Check sheet for the drawn part. Datum: minimum x, y, z corner. Units: mm. Round coordinates to 2 decimals unless told otherwise and drop trailing zeros. Write each loop counter-clockwise with the first axis right and the second up, starting at its lowest first coordinate (ties: lowest second). Pieces come first, ordered by that corner, then holes. Notation, with made-up numbers: M -7.75,-14.5 L 30.25,-14.5 A23 cw 30.25,7.5 Z; hole C 6.5,-30 d11. An arc over 180 degrees is marked long. One line per item, written item: value.
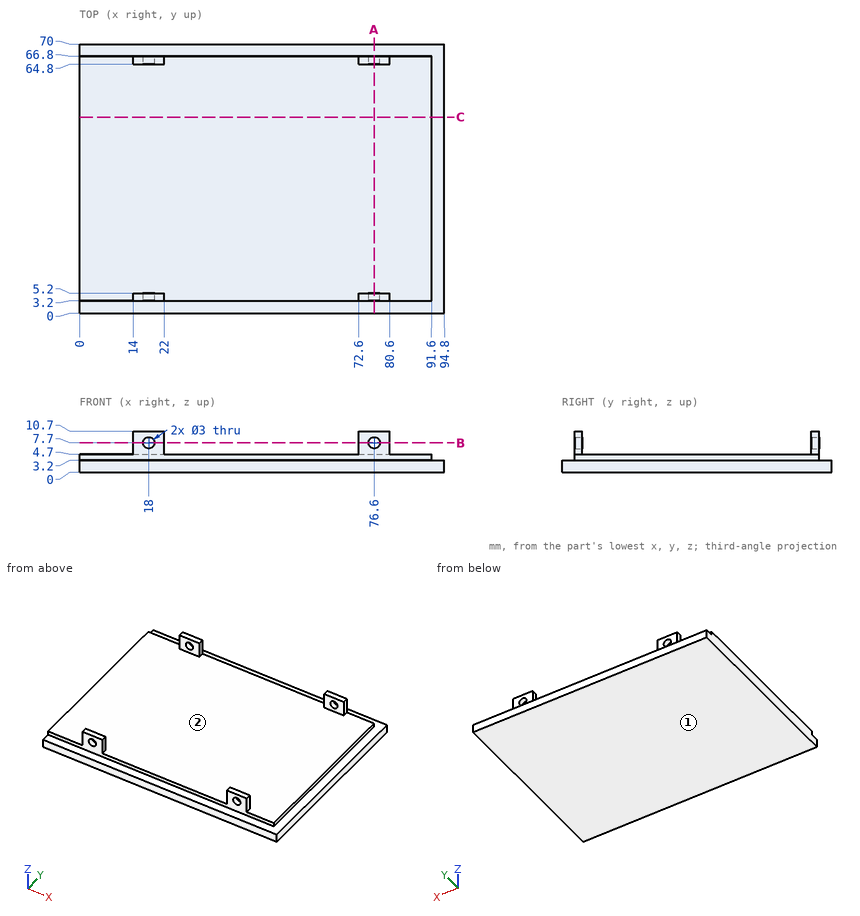
Q1. Sectioned sample at C-C on y = 51. Enter the section's corners in (x, z).
Completed:
outline: M 0,0 L 94.8,0 L 94.8,3.2 L 91.6,3.2 L 91.6,4.7 L 0,4.7 Z
Q2. Scan lines: line 1 (Z direction, x = 76.6, y = 66.3); line 2 (Y direction, x = 15, z = 6.75); line 3 (Z direction, x = 6, y = 54). Record each from-to range of solid material in increasing order. Write a range as [from, to].
Completed:
line 1: [0, 6.2], [9.2, 10.7]
line 2: [3.2, 5.2], [64.8, 66.8]
line 3: [0, 4.7]
Q3. Draft check along Y on the marked faces 1 and 2. Enter one of: pulls with the +Y half, pulls with the -Y half, needs draft (parallel to the pull), parting line crosses it, or undercut.
Completed:
face 1: needs draft
face 2: undercut
Q4. Sectioned sample at A-A on x = 76.6. Enter the section's corners in (y, z), and give its area (3 significant figures).
Completed:
outline: M 0,0 L 70,0 L 70,3.2 L 66.8,3.2 L 66.8,6.2 L 64.8,6.2 L 64.8,4.7 L 5.2,4.7 L 5.2,6.2 L 3.2,6.2 L 3.2,3.2 L 0,3.2 Z; M 3.2,9.2 L 5.2,9.2 L 5.2,10.7 L 3.2,10.7 Z; M 64.8,9.2 L 66.8,9.2 L 66.8,10.7 L 64.8,10.7 Z
area: 331 mm^2
Q5. Depth check by flat-ended pin: P1, Ø3.5, axis at x = 18, z = 7.7, coming from the +Y side; P2, Ø0.6, axis at y = 65.5, z = 7.5, coming from the -X side; P3, Ø1, axis at y = 14.5, z = 4.5, coming from the +X side. Enter the tip coordinate at first touch or a pass-through.
Completed:
P1: y = 66.8
P2: x = 14
P3: x = 91.6
Q6. Sectioned sample at B-B on z = 7.7. State how many separate pieces and enclosed holes the cut face has, and give its area (3 significant figures).
Completed:
separate pieces: 8
enclosed holes: 0
area: 40.0 mm^2
